For this review, use the dimensioned drawing (mm, ordinates from the lowest corner) and the shaded views. Coordinates: 2 decimals unless noted, no trailing zeros. Loops run counter-clockwise (first coordinate to the right, second up) from the corner with the lowest first, then second, coordinate; pieces in that order, holes last. Notation, with made-up numbers: (-35, 36.25) - (11, 36.25) arc R15 ccw to (11, 65.25) - close; hole circle Ø8 at (86, -36.5). An arc over 180 degrees is marked (long way). One line per item, written item: value. Start each with the question number.
1. To check wall thickness, follow line 1 (Y direction, x = 1.5, z = 15); line 2 (Y direction, x = 4.1, z = 16); line 3 (Z direction, x = 3.2, y = 475). State the ranges of each line that lie inside material, in increasing order.
2. We need section B-B, the plane z = 15. Give the boundary of the cut face in (x, y).
3. Insertion check: P1, Ø3, axis at y = 360.5, z = 14, coming from the -X side; P2, Ø13.5, axis at y = 475, z = 15, coming from the +X side; P3, Ø1.5, axis at x = 1.5, z = 23.5, coming from the -Y side; P4, Ø1, axis at x = 3.5, z = 9, coming from the +Y side. Each pin has a flat end and moves straight along its axis. Give the tip position at first contact, or say it passes through.
4. We need section A-A, the plane x = 0.8. Give the boundary of the cut face in (y, z).
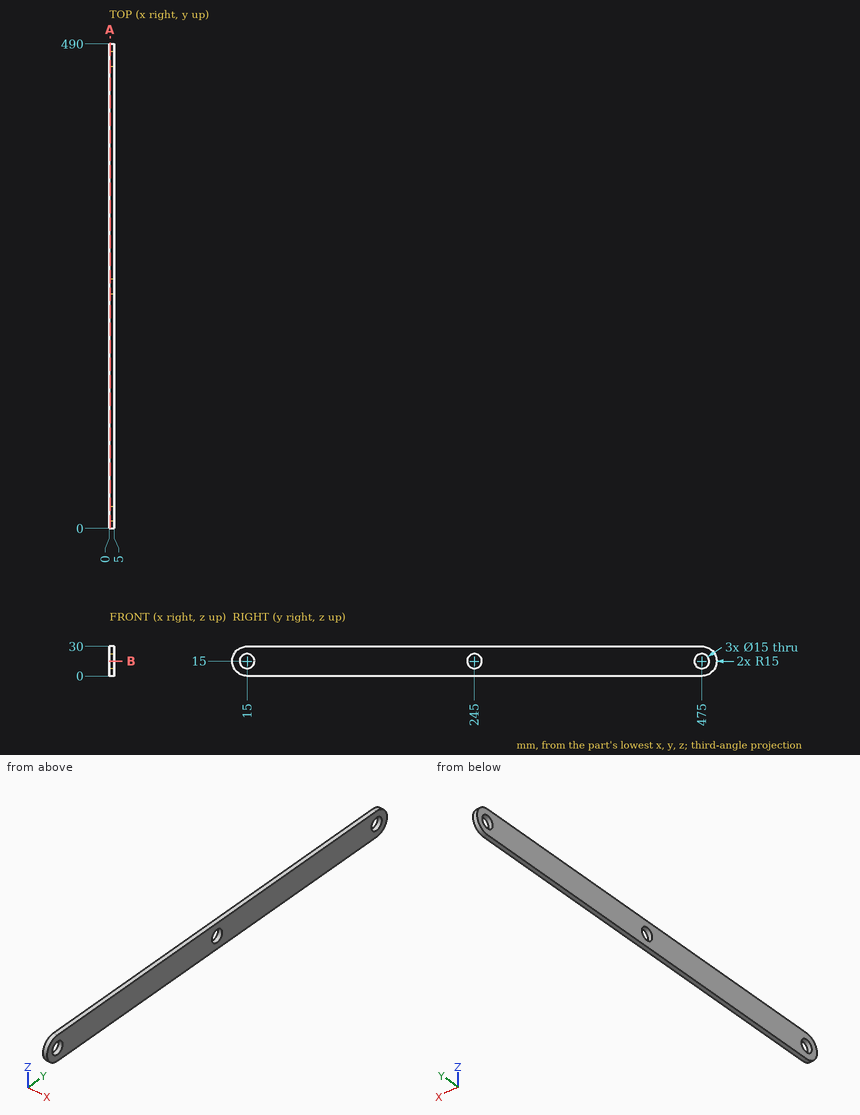
Findings below:
1. line 1: 0 to 7.5, 22.5 to 237.5, 252.5 to 467.5, 482.5 to 490
1. line 2: 0.03 to 7.57, 22.43 to 237.57, 252.43 to 467.57, 482.43 to 489.97
1. line 3: 0 to 7.5, 22.5 to 30
2. outline: (0, 0) - (5, 0) - (5, 7.5) - (0, 7.5) - close; (0, 22.5) - (5, 22.5) - (5, 237.5) - (0, 237.5) - close; (0, 252.5) - (5, 252.5) - (5, 467.5) - (0, 467.5) - close; (0, 482.5) - (5, 482.5) - (5, 490) - (0, 490) - close
3. P1: x = 0
3. P2: through
3. P3: y = 2.16
3. P4: y = 488.96
4. outline: (15, 0) - (475, 0) arc R15 ccw to (475, 30) - (15, 30) arc R15 ccw to start; hole circle Ø15 at (15, 15); hole circle Ø15 at (245, 15); hole circle Ø15 at (475, 15)
